Source: three-view drawing plus pictorial views. Frame: mm from the lowest corner of the part. Coordinates: 2 decimals unless noted, no trailing zeros. Order: outer loops, then holes, each group sorted by start corner. A loop starts at its lowest first (then second) coordinate and runs counter-clockwise, first axis right, second up. Notation, with made-up numbers: (6.5, 65) -> (57.5, 65) arc R36 ccw to (57.5, 103) -> close; hole circle Ø10 at (-5.75, 87.5). An arc over 180 degrees is marked (long way). Use one line per item in the form item = value. Start each with the question number.
1) Ray query, line 1 along X through (y, z) = (0.25, 53); line 2 along Z through (x, y) = (14, 1.1). Return the intervals inside material, ascending.
2) Pin query (flat end, axial travel): pin 1 (0.9 mm diameter, centred on x = 11, y = 1.5, fed in from -Z); pin 2 (8 mm diameter, centred on x = 81, z = 54, fed in from -Y); pin 3 (0.9 mm diameter, centred on x = 97.5, y = 2, fed in from +Z); pin 4 (1.5 mm diameter, centred on y = 1.5, z = 201.5, fed in from +X). Return the tip coordinate at first contact, or that it passes through.
3) Section query A-A on z = 65. Output: boundary loops of the cut face in (x, y), then the cut area to 3 significant figures.
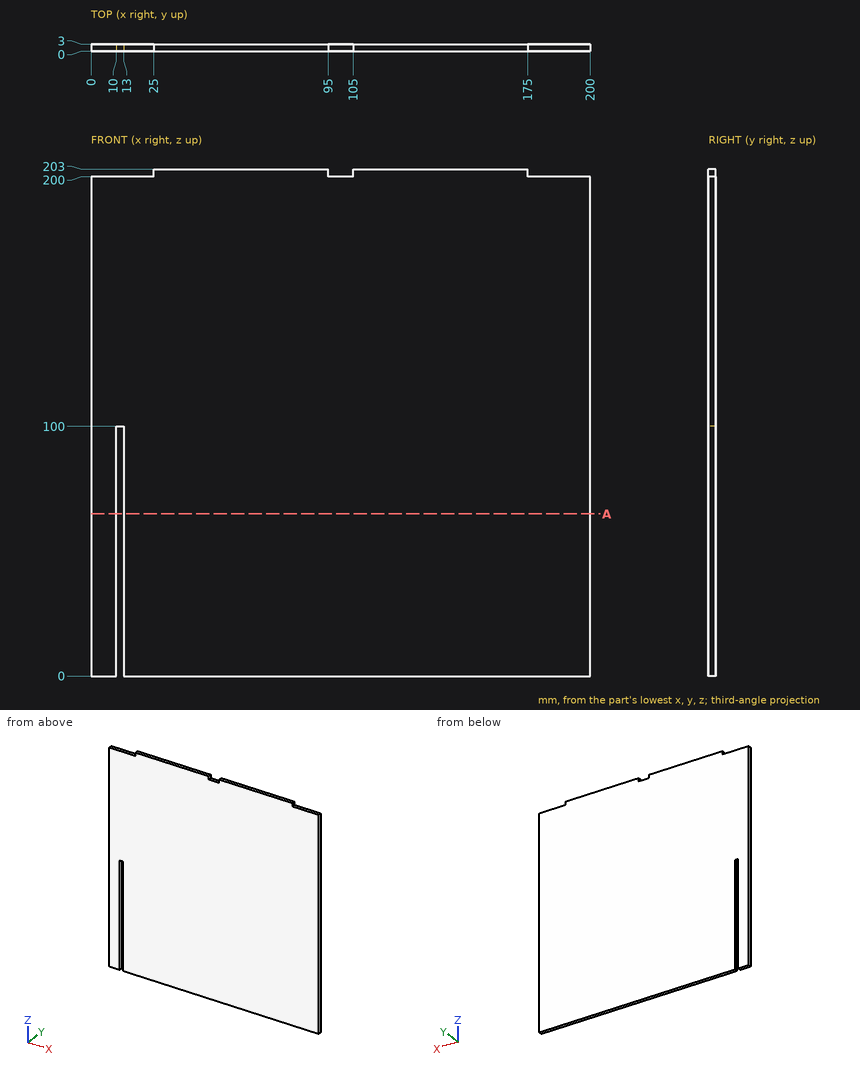
Answers below:
q1.line_1 = 0 to 10, 13 to 200
q1.line_2 = 0 to 200
q2.pin_1 = 100
q2.pin_2 = 0
q2.pin_3 = 200
q2.pin_4 = 175
q3.outline = (0, 0) -> (10, 0) -> (10, 3) -> (0, 3) -> close; (13, 0) -> (200, 0) -> (200, 3) -> (13, 3) -> close
q3.area = 591 mm^2
